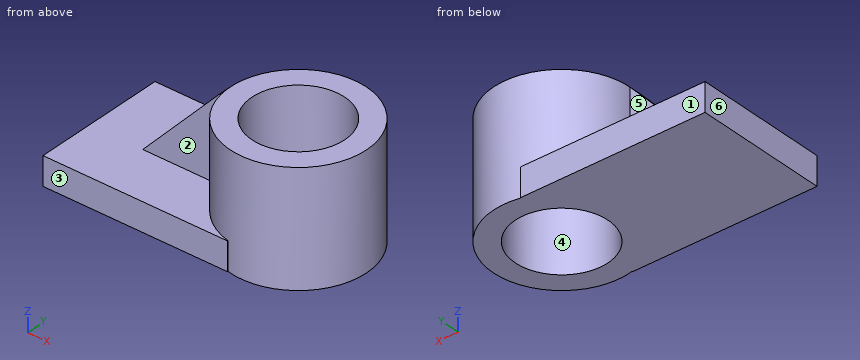
from build123d import *

# Parameters (mm, degrees)
F0_W     = 82.760722
F0_H     = 60.0374
F1_DEPTH = 12.7
F2_R     = 30.531053
F3_DEPTH = 50.8
F5_DEPTH = 5.08
F6_R     = 20.769196
F7_DEPTH = 50.801


with BuildPart() as f1:
    # F0 (on Top) → F1 (new body)
    with BuildSketch(Plane.XY):
        Rectangle(F0_W, F0_H)
    extrude(amount=F1_DEPTH)

    # F2 (on Top) → F3 (join)
    with BuildSketch(Plane.XY):
        with Locations((47.992117, 0.027034)):
            Circle(F2_R)
    extrude(amount=F3_DEPTH)

    # F4 (on Front) → F5 (join)
    with BuildSketch(Plane.XZ):
        Polygon((-17.495457, 12.7), (17.461064, 12.7), (17.461064, 50.8), align=None)
    extrude(amount=F5_DEPTH)

    # F6 (on face) → F7 (cut, through all)
    with BuildSketch(Plane.XY.offset(50.8)):
        with Locations((47.992117, 0.027034)):
            Circle(F6_R)
    extrude(amount=-F7_DEPTH, mode=Mode.SUBTRACT)


solid = f1.part
Design review of the part built by this model. Coordinates are the model's own, in mm. Face numbers are marked on the shaded views. A direction names the side the tool comes from. Round coordinates to 2 decimals unless told otherwise and drop trailing zeros. Write each loop counter-clockwise with the first axis right and the second up, starting at its lowest first coordinate (ties: lowest second). Pieces come first, ordered by that corner, then holes. Notation, with made-up numbers: (-2, 65.25) - (54, 65.25) arc R12 ccw to (54, 71.25) - close; hole circle Ø3 at (-12, 75). An arc over 180 degrees is marked (long way). Return JSON: item names as keys, results as strings. Group by question number.
Item 1: Machinability: for the marked faces 1, 2 and 3, which of the approach directions +Z, -Z, +X, -X, +Y, -Y give a long, thin tool a straight path to every point of the face, cutting with its end or side? Answer none if there is none.
Item 2: We need section C-C on y = 3.5. Write out the cut boundary in (x, z) (3 decimals), and give its area (3 significant figures).
Item 3: We need section A-A on z = 41. Write out the cut boundary in (x, y).
Item 4: Insertion check: P1, Ø6, axis at x = 34, z = 38, coming from the -Y side; P2, Ø14, axis at x = -18.5, z = 3.5, coming from the +Y side; P3, Ø4, axis at x = 6, z = 4.5, coming from the -Y side. Each pin has a flat end and moves straight along its axis. Give the tip position at first contact, or say it passes through.
Item 5: The part is to be moulded in two halves that separate along X. For the marked faces 4, 5 and 6, say which applies: pulls with the +X half, pulls with the -X half, needs draft (parallel to the pull), parting line crosses it, or undercut.
Item 6: We need section D-D on x = -7. Write out the cut boundary in (y, z).
Item 7: For probe 1 along Z at (x, y) = (14.5, 15.5); probe 2 along Y at (x, z) = (15, 17.5); probe 3 along X at (y, z) = (-6, 3.5), list the stretches that pass through material, from the lowest coordinate up. Write a range as [from, to].
Item 8: We need section B-B on x = 50. Write out the cut boundary in (y, z).
Model answer:
{
 "1": {"face 1": "+Z, -Z, -X, +Y", "face 2": "+Z, -X, -Y", "face 3": "+Z, -Z, -X, -Y"},
 "2": {"outline": "(-41.38, 0) - (27.515, 0) - (27.515, 50.8) - (17.659, 50.8) - (17.659, 12.7) - (-41.38, 12.7) - close; (68.469, 0) - (78.325, 0) - (78.325, 50.8) - (68.469, 50.8) - close", "area": "1,750 mm²"},
 "3": {"outline": "(8.47, -5.08) - (17.46, -5.08) - (17.46, 0) - (8.47, 0) - close; circle Ø61.06 at (47.99, 0.03); hole circle Ø41.54 at (47.99, 0.03)"},
 "4": {"P1": "stops at y = -28.46", "P2": "stops at y = 30.02", "P3": "stops at y = -30.02"},
 "5": {"face 4": "undercut", "face 5": "needs draft", "face 6": "pulls with the -X half"},
 "6": {"outline": "(-30.02, 0) - (30.02, 0) - (30.02, 12.7) - (0, 12.7) - (0, 24.14) - (-5.08, 24.14) - (-5.08, 12.7) - (-30.02, 12.7) - close"},
 "7": {"probe 1": "z = [0, 12.7]", "probe 2": "y = [-5.08, 0]", "probe 3": "x = [-41.38, 28.12], [67.87, 77.92]"},
 "8": {"outline": "(-30.44, 0) - (-20.64, 0) - (-20.64, 50.8) - (-30.44, 50.8) - close; (20.7, 0) - (30.49, 0) - (30.49, 50.8) - (20.7, 50.8) - close"}
}
